Input: dimensioned drawing with shaded views. Units: mm. Origin: part minimum x, y, z. A direction names the side the tool comes from. Coordinates: 2 decimals unless noted, no trailing zeros. Loops run counter-clockwise (first coordinate to the right, second up) from the corner with the lowest first, then second, coordinate; pieces in that order, holes last.
Item 1: Contact query for flat-ended pins moving along their axis: P1, Ø5, axis at x = 46.5, y = 38.5, coming from the +Z side; P2, Ø12.5, axis at x = 198, y = 42, coming from the +Z side. Output: stop coordinate, or through.
Item 2: Section A-A on y = 13. Return loops of the section in (x, z), and give its area (3 significant figures).
Item 3: Ray query, line 1 along X through (y, z) = (39, 50); line 2 along Z through (x, y) = (71, 56.5); line 3 along Z through (x, y) = (10, 5). Return the intervals inside material, ascending.
Item 4: Section B-B on z = 41.5. Return loops of the section in (x, y), and give its area (3 significant figures).
Item 5: Section C-C on x = 194. Return loops of the section in (y, z), and give its area (3 significant figures).
Item 6: Reachability of the marked faces 1, 2 and 3 from +Z, -Z, +X, -X, +Y, -Y: full face, straight path, thin tool, end or side. Return the list, or none.
Item 7: Section D-D on x = 29. Return loops of the section in (y, z), and give its area (3 significant figures).
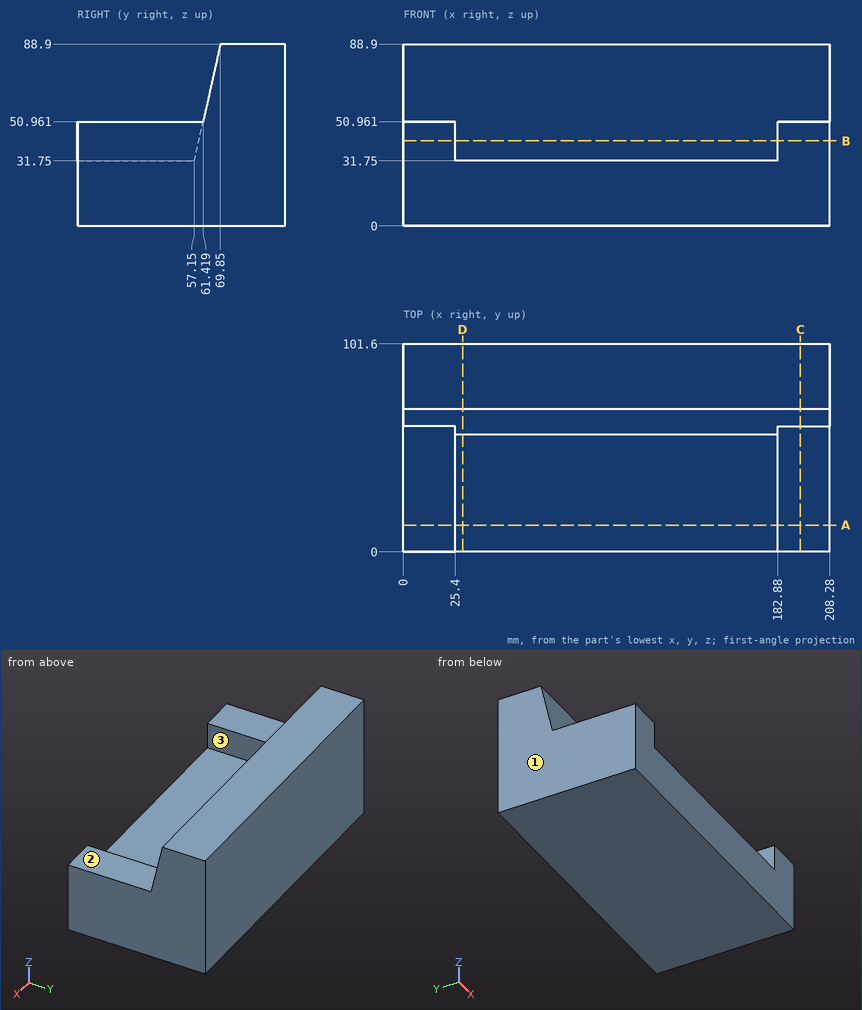
Results found:
1. P1: stops at z = 31.75
1. P2: stops at z = 50.96
2. outline: (0, 0) - (208.28, 0) - (208.28, 50.96) - (182.88, 50.96) - (182.88, 31.75) - (25.4, 31.75) - (25.4, 50.96) - (0, 50.96) - close
2. area: 7,590 mm2
3. line 1: x = 0 to 25.4, 182.88 to 208.28
3. line 2: z = 0 to 31.75
3. line 3: z = 0 to 50.96
4. outline: (0, 0) - (25.4, 0) - (25.4, 59.32) - (182.88, 59.32) - (182.88, 0) - (208.28, 0) - (208.28, 101.6) - (0, 101.6) - close
4. area: 11,800 mm2
5. outline: (0, 0) - (101.6, 0) - (101.6, 88.9) - (69.85, 88.9) - (61.42, 50.96) - (0, 50.96) - close
5. area: 6,540 mm2
6. face 1: +Z, -Z, -X, +Y, -Y
6. face 2: +Z, +X, -X, -Y
6. face 3: +Z, -Y
7. outline: (0, 0) - (101.6, 0) - (101.6, 88.9) - (69.85, 88.9) - (57.15, 31.75) - (0, 31.75) - close
7. area: 5,400 mm2
